```python
from build123d import *

# Parameters (mm, degrees)
BOSS_EXTRUDE1_DEPTH      = 10
BOSS_EXTRUDE2_DEPTH      = 40
BOSS_EXTRUDE2_DEPTH_BACK = 20
CUT_EXTRUDE1_DEPTH       = 61
SKETCH5_W                = 60
SKETCH5_H                = 10
BOSS_EXTRUDE3_DEPTH      = 20
CUT_EXTRUDE2_REACH       = 88
SKETCH6_R                = 6
SKETCH9_W                = 60
SKETCH9_H                = 16
SKETCH9_R                = 3
CUT_EXTRUDE4_DEPTH       = 3
SKETCH10_R               = 3
CUT_EXTRUDE5_DEPTH       = 38


with BuildPart() as part:
    # Sketch1 → Boss-Extrude1 (new body)
    with BuildSketch(Plane(origin=(0, 0, 0), x_dir=(1, 0, 0), z_dir=(0, 1, 0))):
        with BuildLine():
            Line((-30, 0), (-15.411351, 34.300029))
            ThreePointArc((-15.411351, 34.300029), (0, 46), (15.411351, 34.300029))
            Line((15.411351, 34.300029), (30, 0))
            Line((30, 0), (30, -40))
            Line((30, -40), (-30, -40))
            Line((-30, -40), (-30, 0))
        make_face()
    extrude(amount=BOSS_EXTRUDE1_DEPTH)

    # Sketch2 → Boss-Extrude2 (add, two sides)
    with BuildSketch(Plane(origin=(0, 10, 0), x_dir=(1, 0, 0), z_dir=(0, 1, 0))) as boss_extrude2_sk:
        with BuildLine():
            ThreePointArc((15.411351, 34.300029), (0, 46), (-15.411351, 34.300029))
            ThreePointArc((-15.411351, 34.300029), (-2.170066, 14.147845), (16, 30))
            ThreePointArc((16, 30), (15.852155, 32.170066), (15.411351, 34.300029))
        make_face()
    extrude(amount=BOSS_EXTRUDE2_DEPTH)
    extrude(boss_extrude2_sk.sketch, amount=-BOSS_EXTRUDE2_DEPTH_BACK)

    # Sketch3 → Cut-Extrude1 (cut, through all)
    with BuildSketch(Plane(origin=(0, 50, 0), x_dir=(1, 0, 0), z_dir=(0, 1, 0))):
        with BuildLine():
            Line((-3, 44), (3, 44))
            Line((3, 44), (3, 40.583005))
            ThreePointArc((3, 40.583005), (0, 19), (-3, 40.583005))
            Line((-3, 40.583005), (-3, 44))
        make_face()
    extrude(amount=-CUT_EXTRUDE1_DEPTH, mode=Mode.SUBTRACT)

    # Sketch5 → Boss-Extrude3 (add)
    with BuildSketch(Plane(origin=(0, 0, 0), x_dir=(-1, 0, 0), z_dir=(0, -1, 0))):
        with Locations((0, -35)):
            Rectangle(SKETCH5_W, SKETCH5_H)
    extrude(amount=BOSS_EXTRUDE3_DEPTH)

    # Sketch6 → Cut-Extrude2 (cut, up to next)
    with BuildSketch(Plane.XY.offset(40), mode=Mode.PRIVATE) as cut_extrude2_sk1:
        with Locations((16.477302, -10)):
            Circle(SKETCH6_R)
    cut_extrude2_tool1 = extrude(cut_extrude2_sk1.sketch, amount=-CUT_EXTRUDE2_REACH, mode=Mode.PRIVATE) & part.part
    add(cut_extrude2_tool1.solids().sort_by_distance((16.477302, -10, 40))[0], mode=Mode.SUBTRACT)
    # Sketch6 → Cut-Extrude2 (cut, up to next)
    with BuildSketch(Plane.XY.offset(40), mode=Mode.PRIVATE) as cut_extrude2_sk2:
        with Locations((-16.477302, -10)):
            Circle(SKETCH6_R)
    cut_extrude2_tool2 = extrude(cut_extrude2_sk2.sketch, amount=-CUT_EXTRUDE2_REACH, mode=Mode.PRIVATE) & part.part
    add(cut_extrude2_tool2.solids().sort_by_distance((-16.477302, -10, 40))[0], mode=Mode.SUBTRACT)

    # Sketch9 → Cut-Extrude4 (cut)
    with BuildSketch(Plane(origin=(0, 10, 0), x_dir=(1, 0, 0), z_dir=(0, 1, 0))):
        with Locations((0, -18)):
            Rectangle(SKETCH9_W, SKETCH9_H)
        with Locations((0, -18)):
            Circle(SKETCH9_R, mode=Mode.SUBTRACT)
        with Locations((20, -18)):
            Circle(SKETCH9_R, mode=Mode.SUBTRACT)
        with Locations((-20, -18)):
            Circle(SKETCH9_R, mode=Mode.SUBTRACT)
    extrude(amount=-CUT_EXTRUDE4_DEPTH, mode=Mode.SUBTRACT)

    # Sketch10 → Cut-Extrude5 (cut, through all)
    with BuildSketch(Plane(origin=(0, 17, 0), x_dir=(1, 0, 0), z_dir=(0, 1, 0))):
        with Locations((20, -18)):
            Circle(SKETCH10_R)
        with Locations((0, -18)):
            Circle(SKETCH10_R)
        with Locations((-20, -18)):
            Circle(SKETCH10_R)
    extrude(amount=-CUT_EXTRUDE5_DEPTH, mode=Mode.SUBTRACT)


solid = part.part
```
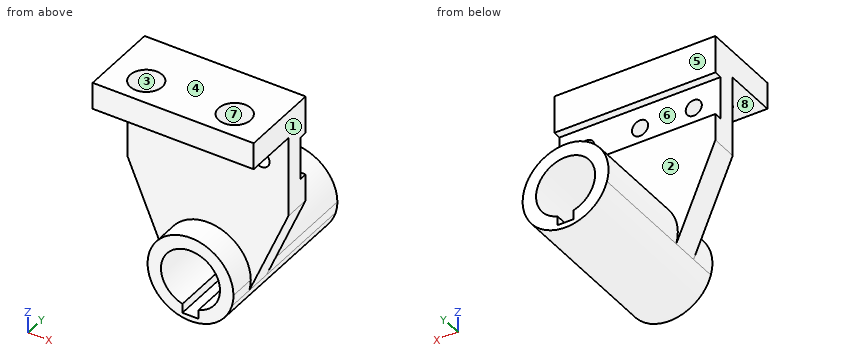
Geometry check sheet. Reference: the model listing, model coordinates, mm. Face numbers are marked on the shaded views. A direction names the side the tool comes from. Round coordinates to 2 decimals unless told otherwise and drop trailing zeros. Order: outer loops, then holes, each group sorted by start corner. A loop starts at its lowest first (then second) coordinate and runs counter-clockwise, first axis right, second up. Notation, with made-up numbers: (-2, 26) - (37, 26) arc R19 cw to (37, 30) - close; hole circle Ø7 at (-2.5, 51.5). An arc over 180 degrees is marked (long way). Use a Markdown table: item, result. Add a question column.
(1) Release check for a two-part mould opening along Y. For the marked faces 1, 2 and 3 record: pulls with the +Y half, pulls with the -Y half, needs draft (parallel to the pull), parting line crosses it, or undercut.
(2) Sectioned sample at D-D, the plane y = -12. Enter the section's corners in (x, z).
(3) Depth check by flat-ended pin: pin 1 (9.5 mm diameter, centred on x = 16.48, y = -10, fed in from +Z); pin 2 (1 mm diameter, centred on y = 1.5, z = -15, fed in from -X); pin 3 (18 mm diameter, centred on x = 11, z = -8.5, fed in from -Y). Enter the tip coordinate at first touch or a pass-through.
(4) Sectioned sample at B-B, the plane y = 34.5. Enter the section's corners in (x, z), and give its area (3 significant figures).
(5) Material ranges on line 1 along X through (y, z) = (4.75, 18); line 2 along Y through (x, z) = (-9, 22.5); line 3 along Y through (x, z) = (-12, 5.5), recorded low to high. Write a range as [from, to].
(6) Tool access check on the marked faces 4, 5, 6, 7 and 8. Record the directions out of +Z, -Z, +X, -X, +Y, -Y that give a thin tool (end or side, any length) a straight path to the whole face; none if there is none.
(7) Sectioned sample at A-A, the plane x = 0. Enter the section's corners in (y, z).
(8) Sectioned sample at C-C, the plane z = 18. Enter the section's corners in (x, y), and give its area (3 significant figures).
Answers below:
| question | item | result |
|---|---|---|
| 1 | face 1 | needs draft |
| 1 | face 2 | pulls with the +Y half |
| 1 | face 3 | undercut |
| 2 | outline | (-30, 30) - (-22.13, 30) - (-22.13, 40) - (-30, 40) - close; (-10.82, 30) - (10.82, 30) - (10.82, 40) - (-10.82, 40) - close; (22.13, 30) - (30, 30) - (30, 40) - (22.13, 40) - close |
| 3 | pin 1 | z = -19.12 |
| 3 | pin 2 | x = -23.83 |
| 3 | pin 3 | y = -10 |
| 4 | outline | (15.41, -34.3) arc R16 ccw to (16, -30) arc R16 ccw (long way) to start; hole (-3, -44) - (3, -44) - (3, -40.58) arc R11 ccw (long way) to (-3, -40.58) - close |
| 4 | area | 405 mm² |
| 5 | line 1 | [-30, -23], [-17, -3], [3, 17], [23, 30] |
| 5 | line 2 | [0, 7] |
| 5 | line 3 | [0, 10] |
| 6 | face 4 | +Z, +X, -X, +Y, -Y |
| 6 | face 5 | +Z, +X, -X, +Y |
| 6 | face 6 | +X, -X, +Y |
| 6 | face 7 | +Z |
| 6 | face 8 | +X, -X, -Y |
| 7 | outline | (-20, 30) - (0, 30) - (0, 21) - (7, 21) - (7, 26) - (10, 26) - (10, 40) - (-20, 40) - close; (-10, -46) - (50, -46) - (50, -44) - (-10, -44) - close; (-10, -19) - (50, -19) - (50, -14) - (10, -14) - (10, 10) - (7, 10) - (7, 15) - (0, 15) - (0, -14) - (-10, -14) - close |
| 8 | outline | (-30, 0) - (-23, 0) - (-23, 7) - (-30, 7) - close; (-17, 0) - (-3, 0) - (-3, 7) - (-17, 7) - close; (3, 0) - (17, 0) - (17, 7) - (3, 7) - close; (23, 0) - (30, 0) - (30, 7) - (23, 7) - close |
| 8 | area | 294 mm² |
